```python
from build123d import *

# Parameters (mm, degrees)
SKETCH1_W           = 30
SKETCH1_H           = 20
SKETCH1_H_2         = 2.5
SKETCH1_W_2         = 16
SKETCH1_W_3         = 7
SKETCH1_H_3         = 10.6
BOSS_EXTRUDE1_DEPTH = 6
SKETCH1_3_W         = 7
SKETCH1_3_H         = 2.5
SKETCH1_3_W_2       = 16
SKETCH1_3_W_3       = 30
BOSS_EXTRUDE2_DEPTH = 12
SKETCH3_R           = 1.5
CUT_EXTRUDE2_DEPTH  = 16
CUT_EXTRUDE1_DEPTH  = 38.976966704
SKETCH5_W           = 5
SKETCH5_H           = 12
SKETCH5_W_2         = 30
SKETCH5_H_2         = 2.5
BOSS_EXTRUDE3_DEPTH = 9
SKETCH6_R           = 1.5
CUT_EXTRUDE4_DEPTH  = 16.99


with BuildPart() as part:
    # Sketch1 → Boss-Extrude1 (new body)
    with BuildSketch(Plane(origin=(0, 0, 0), x_dir=(1, 0, 0), z_dir=(0, 1, 0))):
        with Locations((-15, -10)):
            Rectangle(SKETCH1_W, SKETCH1_H)
        with Locations((-15, -21.25)):
            Rectangle(SKETCH1_W, SKETCH1_H_2)
        with Locations((-15, 1.25)):
            Rectangle(SKETCH1_W_2, SKETCH1_H_2)
        with Locations((-3.5, 1.25)):
            Rectangle(SKETCH1_W_3, SKETCH1_H_2)
        with Locations((-3.5, 7.8)):
            Rectangle(SKETCH1_W_3, SKETCH1_H_3)
        with Locations((-3.5, 14.35)):
            Rectangle(SKETCH1_W_3, SKETCH1_H_2)
        with Locations((-15, 14.35)):
            Rectangle(SKETCH1_W_2, SKETCH1_H_2)
        with Locations((-26.5, 14.35)):
            Rectangle(SKETCH1_W_3, SKETCH1_H_2)
        with Locations((-26.5, 7.8)):
            Rectangle(SKETCH1_W_3, SKETCH1_H_3)
        with Locations((-26.5, 1.25)):
            Rectangle(SKETCH1_W_3, SKETCH1_H_2)
    extrude(amount=BOSS_EXTRUDE1_DEPTH)

    # Sketch1_3 → Boss-Extrude2 (add)
    with BuildSketch(Plane(origin=(0, 0, 0), x_dir=(1, 0, 0), z_dir=(0, 1, 0))):
        with Locations((-3.5, 1.25)):
            Rectangle(SKETCH1_3_W, SKETCH1_3_H)
        with Locations((-15, 1.25)):
            Rectangle(SKETCH1_3_W_2, SKETCH1_3_H)
        with Locations((-15, -21.25)):
            Rectangle(SKETCH1_3_W_3, SKETCH1_3_H)
        with Locations((-26.5, 1.25)):
            Rectangle(SKETCH1_3_W, SKETCH1_3_H)
    extrude(amount=BOSS_EXTRUDE2_DEPTH)

    # Sketch3 → Cut-Extrude2 (cut)
    with BuildSketch(Plane(origin=(0, 0, -15.6), x_dir=(-1, 0, 0), z_dir=(0, 0, -1))):
        with Locations((15, 3)):
            Circle(SKETCH3_R)
    extrude(amount=-CUT_EXTRUDE2_DEPTH, mode=Mode.SUBTRACT)

    # Sketch2 → Cut-Extrude1 (cut, through all)
    with BuildSketch(Plane(origin=(0, 6, 0), x_dir=(1, 0, 0), z_dir=(0, 1, 0))):
        with BuildLine():
            ThreePointArc((-13, -10), (-15, -8), (-17, -10))
            Line((-17, -10), (-13, -10))
        make_face()
        with BuildLine():
            Line((-13, -10), (-17, -10))
            ThreePointArc((-17, -10), (-15, -12), (-13, -10))
        make_face()
    extrude(amount=-CUT_EXTRUDE1_DEPTH, mode=Mode.SUBTRACT)

    # Sketch5 → Boss-Extrude3 (add)
    with BuildSketch(Plane.XZ):
        with Locations((-27.5, 28.5)):
            Rectangle(SKETCH5_W, SKETCH5_H)
        with Locations((-15, 35.75)):
            Rectangle(SKETCH5_W_2, SKETCH5_H_2)
        with Locations((-2.5, 28.5)):
            Rectangle(SKETCH5_W, SKETCH5_H)
    extrude(amount=-BOSS_EXTRUDE3_DEPTH)

    # Sketch6 → Cut-Extrude4 (cut)
    with BuildSketch(Plane.XY.offset(37)):
        with Locations((-15, 4.5)):
            Circle(SKETCH6_R)
    extrude(amount=-CUT_EXTRUDE4_DEPTH, mode=Mode.SUBTRACT)


solid = part.part
```
Verification items for the finished model (mm, model axes). A direction names the side the tool comes from. Coordinates: 2 decimals unless noted, no trailing zeros. Order: outer loops, then holes, each group sorted by start corner. A loop starts at its lowest first (then second) coordinate and runs counter-clockwise, first axis right, second up. Notation, with made-up numbers: (-34.5, -22.5) -> (-0.5, -22.5) arc R26 cw to (-0.5, 1.5) -> close; hole circle Ø3 at (73, 33.25). An arc over 180 degrees is marked (long way). Put each result on its own line as item: value. Start each with the question number.
1) Release check for a two-part mould opening along X. For faces 6 (the flat face through (-15, 3, 0.4)), 7 (the flat face through (-19, 0, 11)), 8 (the flat face through (0, 5, 11)) record: pulls with the +X half, pulls with the -X half, needs draft (parallel to the pull), parting line crosses it, or undercut.
2) Cross-section at D-D (y = 1). Enter the section's corners in (x, z).
3) Go/stop test with flat-tipped pins: pin 1 (5 mm diameter, centred on x = -21.5, y = 9, fed in from -Z); pin 2 (3 mm diameter, centred on x = -20, z = -8.5, fed in from +Y); pin 3 (4 mm diameter, centred on x = -19, z = -12, fed in from +Y). Record where each tip stops, or that it passes through.
4) Cross-section at A-A (y = 7.5). Enter the section's corners in (x, z).
5) Material ranges on L1, parallel to Z at x = -8.5, y = 5.25; L2, parallel to Z at x = -19.5, y = 6.5; L3, parallel to X at y = 3.5, z = -7, recorded low to high.
6) Cross-section at B-B (x = -8.25). Enter the section's corners in (y, z).
7) Cross-section at C-C (z = 10). Enter the section's corners in (x, y).
8) Tool access check on faces 1 (the cylindrical face through (-16.5, 4.57, 21.27)), 2 (the flat face through (-15, 7, -2.5)), 3 (the flat face through (-15.1, 6.4, 34.5)), 4 (the flat face through (-15, 9, 20)), 5 (the flat face through (-19, 9, 35)). Record the directions out of +Z, -Z, +X, -X, +Y, -Y that give a thin tool (end or side, any length) a straight path to the whole face; none if there is none.
Geometry check:
1. face 6: undercut
1. face 7: needs draft
1. face 8: pulls with the +X half
2. outline: (-30, -15.6) -> (0, -15.6) -> (0, 37) -> (-30, 37) -> close; hole (-25, 22.5) -> (-5, 22.5) -> (-5, 34.5) -> (-25, 34.5) -> close; hole (-23, -13.1) -> (-7, -13.1) -> (-7, -2.5) -> (-23, -2.5) -> close; hole circle Ø4 at (-15, 10)
3. pin 1: stops at z = -2.5
3. pin 2: passes through
3. pin 3: stops at y = 6
4. outline: (-30, -2.5) -> (0, -2.5) -> (0, 0) -> (-30, 0) -> close; (-30, 20) -> (0, 20) -> (0, 37) -> (-30, 37) -> close; hole (-25, 22.5) -> (-5, 22.5) -> (-5, 34.5) -> (-25, 34.5) -> close
5. L1: z = -15.6 to -13.1, -2.5 to 22.5, 34.5 to 37
5. L2: z = -2.5 to 0, 20 to 22.5, 34.5 to 37
5. L3: x = -30 to -23, -7 to 0
6. outline: (0, -15.6) -> (6, -15.6) -> (6, -13.1) -> (0, -13.1) -> close; (0, -2.5) -> (12, -2.5) -> (12, 0) -> (6, 0) -> (6, 20) -> (12, 20) -> (12, 22.5) -> (0, 22.5) -> close; (0, 34.5) -> (9, 34.5) -> (9, 37) -> (0, 37) -> close
7. outline: (-30, 0) -> (-17, 0) -> (-17, 6) -> (-30, 6) -> close; (-13, 0) -> (0, 0) -> (0, 6) -> (-13, 6) -> close
8. face 1: +Z
8. face 2: +Y
8. face 3: +Y, -Y
8. face 4: +X, -X, +Y
8. face 5: +Z, +X, -X, +Y
